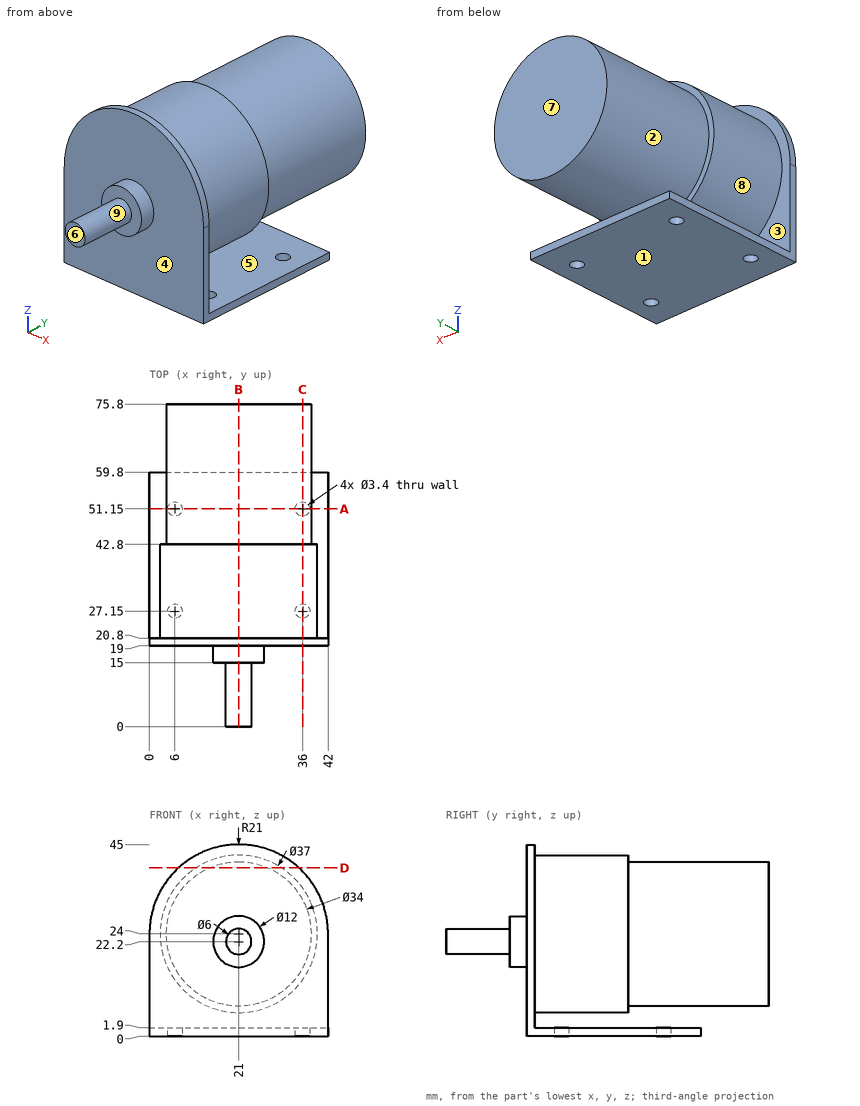
The figure shows three views and two pictorial views of one solid part (mm, origin at its lowest corner). Answer the questions. A direction names the side the tool comes from. Round coordinates to 2 decimals unless told otherwise and drop trailing zeros. Write each loop counter-clockwise with the first axis right and the second up, starting at its lowest first coordinate (ties: lowest second). Pieces come first, ordered by that corner, then holes. Notation, with made-up numbers: M -10.75,89 L -3.75,89 A29 cw -3.75,117 Z; hole C -20,-5 d10. An arc over 180 degrees is marked long. Use a Markdown table: item, result.
1) The part is cut by section C-C on x = 36. Give the vertices of the cut face in (y, z).
Taken from the geometry:
| item | result |
|---|---|
| outline | M 19,0 L 25.45,0 L 25.45,1.9 L 20.8,1.9 L 20.8,13.17 L 42.8,13.17 L 42.8,16 L 75.8,16 L 75.8,32 L 42.8,32 L 42.8,34.83 L 20.8,34.83 L 20.8,38.7 L 19,38.7 Z; M 28.85,0 L 49.45,0 L 49.45,1.9 L 28.85,1.9 Z; M 52.85,0 L 59.8,0 L 59.8,1.9 L 52.85,1.9 Z |
2) The part is cut by section D-D on z = 39.5. Give the vertices of the cut face in (x, y), plus the area to 3 significant figures.
Taken from the geometry:
| item | result |
|---|---|
| outline | M 6.83,19 L 35.17,19 L 35.17,20.8 L 31.1,20.8 L 31.1,42.8 L 27.98,42.8 L 27.98,75.8 L 14.02,75.8 L 14.02,42.8 L 10.9,42.8 L 10.9,20.8 L 6.83,20.8 Z |
| area | 956 mm2 |
3) Which of the six approach directions +Z, -Z, +X, -X, +Y, -Y give full straight-line access (tool end or side, diameter ignored) to the marked faces 5, 6, 7, 8 and 9?
Taken from the geometry:
| item | result |
|---|---|
| face 5 | +X, -X, +Y |
| face 6 | +Z, -Z, +X, -X, -Y |
| face 7 | +Z, -Z, +X, -X, +Y |
| face 8 | +Y |
| face 9 | -Y |
4) The part is cut by section B-B on x = 21. Give the vertices of the cut face in (y, z), plus the area to 3 significant figures.
Taken from the geometry:
| item | result |
|---|---|
| outline | M 0,19.2 L 15,19.2 L 15,16.2 L 19,16.2 L 19,0 L 59.8,0 L 59.8,1.9 L 20.8,1.9 L 20.8,5.5 L 42.8,5.5 L 42.8,7 L 75.8,7 L 75.8,41 L 42.8,41 L 42.8,42.5 L 20.8,42.5 L 20.8,45 L 19,45 L 19,28.2 L 15,28.2 L 15,25.2 L 0,25.2 Z |
| area | 2,230 mm2 |
5) Consider line 1 (Y direction, x = 6, z = 0.6); line 2 (Z direction, x = 21.5, y = 36.5); line 3 (Y direction, x = 25, z = 9). Determine where each line is inside the solid, lowest interval first. Write a range as [from, to].
Taken from the geometry:
| item | result |
|---|---|
| line 1 | y = [19, 25.45], [28.85, 49.45], [52.85, 59.8] |
| line 2 | z = [0, 1.9], [5.51, 42.49] |
| line 3 | y = [19, 75.8] |
6) The part is cut by section A-A on y = 51.15. Give the vertices of the cut face in (x, z).
Taken from the geometry:
| item | result |
|---|---|
| outline | M 0,0 L 4.3,0 L 4.3,1.9 L 0,1.9 Z; C 21,24 d34; M 7.7,0 L 34.3,0 L 34.3,1.9 L 7.7,1.9 Z; M 37.7,0 L 42,0 L 42,1.9 L 37.7,1.9 Z |
7) Flat-ended cylindrical pins translate along their axes: pin 1 (2 mm diameter, centred on x = 30.5, y = 51, fed in from +Z); pin 2 (12 mm diameter, centred on x = 34.5, z = 40, fed in from -Y); pin 3 (3 mm diameter, centred on x = 36, y = 27.15, fed in from +Z). Find the tip coordinate at first contact, or state that the pin passes through.
Taken from the geometry:
| item | result |
|---|---|
| pin 1 | stops at z = 38.72 |
| pin 2 | stops at y = 19 |
| pin 3 | stops at z = 36.65 |
8) Determine the mould class of the marked faces 1, 2, 3 and 4 for opening direction Z: pulls with the +Z half, pulls with the -Z half, needs draft (parallel to the pull), parting line crosses it, or undercut.
Taken from the geometry:
| item | result |
|---|---|
| face 1 | pulls with the -Z half |
| face 2 | undercut |
| face 3 | undercut |
| face 4 | needs draft |
